Could you check a few things on this model? Use its own coordinates, in mm. A direction names the side the tool comes from. Give positions to 0.01 mm unless a question says otherwise; leave off trailing zeros. Order: outer loops, then holes, each group sorted by start corner. A loop starts at its lowest first (then second) coordinate and runs counter-clockwise, first axis right, second up. Notation, with made-up numbers: M -2,-1 L 43,-1 A33 ccw 43,31 Z; hole C 62.5,-30 d2. An arc over 180 degrees is marked long. Use a Markdown table: item, result. Add a question column.
Item 1: For faces 4 (the face through (-3, 6, -22)), 5 (the face through (-3.5, 5, -22)), which set-ups out of +Z, -Z, +X, -X, +Y, -Y let a thin tool reach every point of the face, with its end or its side?
Item 2: If we mould it in two halves opening along X, with no side actions, what happens to faces 1 (the face through (-5, 3, -45.5)), 2 (the face through (-9.5, 3, -22)), 3 (the face through (-5, 5, -4.25))? For each: released by +X, released by -X, zero draft, split by the parting line, or undercut.
Item 3: If I drill on L1, parallel to X at y = 4.5, z = -40.5; L2, parallel to Z at x = -4.25, y = 4.3; L3, parallel to Y at x = -5, z = -22.5, over which ranges is the centre line in solid material (lowest first)? Write a range as from..to.
Item 4: Suppose I cut it at A-A on x = -5.5. Write out the boundary of the cut face in (y, z).
Item 5: Suppose I cut it at B-B on z = -31. Write out the boundary of the cut face in (x, y).
Autodesk Inventor part; units mm, degrees
ref_plane "YZ Plane" through (0, 0, 0) normal (1, 0, 0) x (0, 1, 0)
ref_plane "XZ Plane" through (0, 0, 0) normal (0, 1, 0) x (-1, 0, 0)
ref_plane "XY Plane" through (0, 0, 0) normal (0, 0, 1) x (1, 0, 0)
sketch "Sketch1" plane through (0, 0, 0) normal (0, 1, 0) x (-1, 0, 0)
  line L0 (0, 0) -> (9.5, 0)
  line L1 (9.5, 0) -> (9.5, -45.5)
  line L2 (9.5, -45.5) -> (0, -45.5)
  line L3 (0, -45.5) -> (0, 0)
  dimension "d0" = 9.5
  dimension "d1" = 45.5
extrude "Extrusion1" add sketch "Sketch1" along normal blind 6
sketch "Sketch2" plane through (0, 6, 0) normal (0, 1, 0) x (1, 0, 0)
  line L0 (-9.5, 0) -> (0, 0)
  line L1 (0, 0) -> (0, 45.5)
  line L2 (0, 45.5) -> (-9.5, 45.5)
  line L3 (-9.5, 45.5) -> (-9.5, 0)
  line L4 (-6, 4.25) -> (-3.5, 4.25)
  line L5 (-3.5, 4.25) -> (-3.5, 41.25)
  line L6 (-3.5, 41.25) -> (-6, 41.25)
  line L7 (-6, 41.25) -> (-6, 4.25)
  line L8 (-4.75, 41.25) -> (-4.75, 45.5)
  line L9 (0, 45.5) -> (-9.5, 45.5)
  line L10 (-6, 22.75) -> (-9.5, 22.75)
  line L11 (-9.5, 45.5) -> (-9.5, 0)
  line L12 (-4.75, 4.25) -> (-4.75, 0)
  line L13 (-9.5, 0) -> (0, 0)
  line L14 (-3.5, 22.75) -> (0, 22.75)
  dimension "d4" = 2.5
  dimension "d5" = 37
extrude "Extrusion2" cut sketch "Sketch2" against normal blind 2 contours L4 L7 L6 L5
properties part number "Linear Resistor Body"
Findings below:
| question | item | result |
|---|---|---|
| 1 | face 4 | +Z, -Z, +X, -X, +Y |
| 1 | face 5 | +Y |
| 2 | face 1 | zero draft |
| 2 | face 2 | released by -X |
| 2 | face 3 | undercut |
| 3 | L1 | x = -9.5..-6, -3.5..0 |
| 3 | L2 | z = -45.5..-41.25, -4.25..0 |
| 3 | L3 | y = 0..4 |
| 4 | outline | M 0,-45.5 L 6,-45.5 L 6,-41.25 L 4,-41.25 L 4,-4.25 L 6,-4.25 L 6,0 L 0,0 Z |
| 5 | outline | M -9.5,0 L 0,0 L 0,6 L -3.5,6 L -3.5,4 L -6,4 L -6,6 L -9.5,6 Z |
